```python
from build123d import *

# Parameters (mm, degrees)
SKETCH1_R           = 1.55
SKETCH1_W           = 57.8
SKETCH1_H           = 30
SKETCH1_W_2         = 22
SKETCH1_W_3         = 30
BOSS_EXTRUDE1_DEPTH = 10
FILLET2_R           = 8
CHAMFER1_SIZE       = 1
SKETCH2_R           = 3.25
CUT_EXTRUDE1_DEPTH  = 3
CUT_EXTRUDE2_DEPTH  = 137.363814848
CHAMFER2_SIZE       = 1


with BuildPart() as part:
    # Sketch1 → Boss-Extrude1 (new body)
    # profile 1 of 9: a face of its own
    with BuildSketch(Plane.XY):
        Polygon((-25, -31.5), (-25, -41.5), (25, -41.5), (25, -31.5), (25, -1.5), (25, 8.5), (-25, 8.5), (-25, -1.5), align=None)
        with Locations((0, -33)):
            Circle(SKETCH1_R, mode=Mode.SUBTRACT)
        Circle(SKETCH1_R, mode=Mode.SUBTRACT)
    # profile 2 of 9: a face of its own
    with BuildSketch(Plane.XY):
        with Locations((-53.9, -16.5)):
            Rectangle(SKETCH1_W, SKETCH1_H)
    # profile 3 of 9: a face of its own
    with BuildSketch(Plane.XY):
        with Locations((36, -16.5)):
            Rectangle(SKETCH1_W_2, SKETCH1_H)
    # profile 4 of 9: a face of its own
    with BuildSketch(Plane.XY):
        with Locations((-97.8, -16.5)):
            Rectangle(SKETCH1_W_3, SKETCH1_H)
        with BuildLine():
            Line((-99.8, -24.6), (-99.8, -23.6))
            Line((-99.8, -23.6), (-99.267140075, -23.6))
            ThreePointArc((-99.267140075, -23.6), (-98.896015511, -23.003984489), (-98.3, -22.632859925))
            Line((-98.3, -22.632859925), (-98.3, -22.1))
            Line((-98.3, -22.1), (-97.3, -22.1))
            Line((-97.3, -22.1), (-97.3, -22.632859925))
            ThreePointArc((-97.3, -22.632859925), (-96.703984489, -23.003984489), (-96.332859925, -23.6))
            Line((-96.332859925, -23.6), (-95.8, -23.6))
            Line((-95.8, -23.6), (-95.8, -24.6))
            Line((-95.8, -24.6), (-96.332859925, -24.6))
            ThreePointArc((-96.332859925, -24.6), (-96.703984489, -25.196015511), (-97.3, -25.567140075))
            Line((-97.3, -25.567140075), (-97.3, -26.1))
            Line((-97.3, -26.1), (-98.3, -26.1))
            Line((-98.3, -26.1), (-98.3, -25.567140075))
            ThreePointArc((-98.3, -25.567140075), (-98.896015511, -25.196015511), (-99.267140075, -24.6))
            Line((-99.267140075, -24.6), (-99.8, -24.6))
        make_face(mode=Mode.SUBTRACT)
        with BuildLine():
            Line((-97.3, -10.9), (-98.3, -10.9))
            Line((-98.3, -10.9), (-98.3, -10.367140075))
            ThreePointArc((-98.3, -10.367140075), (-98.896015511, -9.996015511), (-99.267140075, -9.4))
            Line((-99.267140075, -9.4), (-99.8, -9.4))
            Line((-99.8, -9.4), (-99.8, -8.4))
            Line((-99.8, -8.4), (-99.267140075, -8.4))
            ThreePointArc((-99.267140075, -8.4), (-98.896015511, -7.803984489), (-98.3, -7.432859925))
            Line((-98.3, -7.432859925), (-98.3, -6.9))
            Line((-98.3, -6.9), (-97.3, -6.9))
            Line((-97.3, -6.9), (-97.3, -7.432859925))
            ThreePointArc((-97.3, -7.432859925), (-96.703984489, -7.803984489), (-96.332859925, -8.4))
            Line((-96.332859925, -8.4), (-95.8, -8.4))
            Line((-95.8, -8.4), (-95.8, -9.4))
            Line((-95.8, -9.4), (-96.332859925, -9.4))
            ThreePointArc((-96.332859925, -9.4), (-96.703984489, -9.996015511), (-97.3, -10.367140075))
            Line((-97.3, -10.367140075), (-97.3, -10.9))
        make_face(mode=Mode.SUBTRACT)
    # profile 5 of 9: a face of its own
    with BuildSketch(Plane.XY):
        with Locations((62, -16.5)):
            Rectangle(SKETCH1_W_3, SKETCH1_H)
        with BuildLine():
            Line((55.867140075, -23.6), (56.4, -23.6))
            Line((56.4, -23.6), (56.4, -24.6))
            Line((56.4, -24.6), (55.867140075, -24.6))
            ThreePointArc((55.867140075, -24.6), (55.496015511, -25.196015511), (54.9, -25.567140075))
            Line((54.9, -25.567140075), (54.9, -26.1))
            Line((54.9, -26.1), (53.9, -26.1))
            Line((53.9, -26.1), (53.9, -25.567140075))
            ThreePointArc((53.9, -25.567140075), (53.303984489, -25.196015511), (52.932859925, -24.6))
            Line((52.932859925, -24.6), (52.4, -24.6))
            Line((52.4, -24.6), (52.4, -23.6))
            Line((52.4, -23.6), (52.932859925, -23.6))
            ThreePointArc((52.932859925, -23.6), (53.303984489, -23.003984489), (53.9, -22.632859925))
            Line((53.9, -22.632859925), (53.9, -22.1))
            Line((53.9, -22.1), (54.9, -22.1))
            Line((54.9, -22.1), (54.9, -22.632859925))
            ThreePointArc((54.9, -22.632859925), (55.496015511, -23.003984489), (55.867140075, -23.6))
        make_face(mode=Mode.SUBTRACT)
        with BuildLine():
            Line((67.6, -24.6), (67.6, -23.6))
            Line((67.6, -23.6), (68.132859925, -23.6))
            ThreePointArc((68.132859925, -23.6), (68.503984489, -23.003984489), (69.1, -22.632859925))
            Line((69.1, -22.632859925), (69.1, -22.1))
            Line((69.1, -22.1), (70.1, -22.1))
            Line((70.1, -22.1), (70.1, -22.632859925))
            ThreePointArc((70.1, -22.632859925), (70.696015511, -23.003984489), (71.067140075, -23.6))
            Line((71.067140075, -23.6), (71.6, -23.6))
            Line((71.6, -23.6), (71.6, -24.6))
            Line((71.6, -24.6), (71.067140075, -24.6))
            ThreePointArc((71.067140075, -24.6), (70.696015511, -25.196015511), (70.1, -25.567140075))
            Line((70.1, -25.567140075), (70.1, -26.1))
            Line((70.1, -26.1), (69.1, -26.1))
            Line((69.1, -26.1), (69.1, -25.567140075))
            ThreePointArc((69.1, -25.567140075), (68.503984489, -25.196015511), (68.132859925, -24.6))
            Line((68.132859925, -24.6), (67.6, -24.6))
        make_face(mode=Mode.SUBTRACT)
        with BuildLine():
            Line((56.4, -8.4), (56.4, -9.4))
            Line((56.4, -9.4), (55.867140075, -9.4))
            ThreePointArc((55.867140075, -9.4), (55.496015511, -9.996015511), (54.9, -10.367140075))
            Line((54.9, -10.367140075), (54.9, -10.9))
            Line((54.9, -10.9), (53.9, -10.9))
            Line((53.9, -10.9), (53.9, -10.367140075))
            ThreePointArc((53.9, -10.367140075), (53.303984489, -9.996015511), (52.932859925, -9.4))
            Line((52.932859925, -9.4), (52.4, -9.4))
            Line((52.4, -9.4), (52.4, -8.4))
            Line((52.4, -8.4), (52.932859925, -8.4))
            ThreePointArc((52.932859925, -8.4), (53.303984489, -7.803984489), (53.9, -7.432859925))
            Line((53.9, -7.432859925), (53.9, -6.9))
            Line((53.9, -6.9), (54.9, -6.9))
            Line((54.9, -6.9), (54.9, -7.432859925))
            ThreePointArc((54.9, -7.432859925), (55.496015511, -7.803984489), (55.867140075, -8.4))
            Line((55.867140075, -8.4), (56.4, -8.4))
        make_face(mode=Mode.SUBTRACT)
        with BuildLine():
            Line((70.1, -10.9), (69.1, -10.9))
            Line((69.1, -10.9), (69.1, -10.367140075))
            ThreePointArc((69.1, -10.367140075), (68.503984489, -9.996015511), (68.132859925, -9.4))
            Line((68.132859925, -9.4), (67.6, -9.4))
            Line((67.6, -9.4), (67.6, -8.4))
            Line((67.6, -8.4), (68.132859925, -8.4))
            ThreePointArc((68.132859925, -8.4), (68.503984489, -7.803984489), (69.1, -7.432859925))
            Line((69.1, -7.432859925), (69.1, -6.9))
            Line((69.1, -6.9), (70.1, -6.9))
            Line((70.1, -6.9), (70.1, -7.432859925))
            ThreePointArc((70.1, -7.432859925), (70.696015511, -7.803984489), (71.067140075, -8.4))
            Line((71.067140075, -8.4), (71.6, -8.4))
            Line((71.6, -8.4), (71.6, -9.4))
            Line((71.6, -9.4), (71.067140075, -9.4))
            ThreePointArc((71.067140075, -9.4), (70.696015511, -9.996015511), (70.1, -10.367140075))
            Line((70.1, -10.367140075), (70.1, -10.9))
        make_face(mode=Mode.SUBTRACT)
    # profile 6 of 9: a face of its own
    with BuildSketch(Plane.XY):
        with BuildLine():
            Line((77, -31.5), (47, -31.5))
            ThreePointArc((47, -31.5), (62, -46.5), (77, -31.5))
        make_face()
    # profile 7 of 9: a face of its own
    with BuildSketch(Plane.XY):
        with BuildLine():
            ThreePointArc((-112.8, -1.5), (-127.8, -16.5), (-112.8, -31.5))
            Line((-112.8, -31.5), (-112.8, -1.5))
        make_face()
    # profile 8 of 9: a face of its own
    with BuildSketch(Plane.XY):
        with BuildLine():
            ThreePointArc((77, -1.5), (62, 13.5), (47, -1.5))
            Line((47, -1.5), (77, -1.5))
        make_face()
    # profile 9 of 9: a face of its own
    with BuildSketch(Plane.XY):
        with BuildLine():
            Line((77, -1.5), (77, -31.5))
            ThreePointArc((77, -31.5), (92, -16.5), (77, -1.5))
        make_face()
    extrude(amount=BOSS_EXTRUDE1_DEPTH)

    # Fillet2
    fillet2_edges = [part.edges().sort_by_distance(p)[0] for p in [
        (-25, -1.5, 5),
        (25, -1.5, 5),
        (25, -31.5, 5),
        (-25, -31.5, 5),
    ]]
    fillet(fillet2_edges, radius=FILLET2_R)

    # Chamfer1
    chamfer1_edges = [part.edges().sort_by_distance(p)[0] for p in [
        (-127.8, -16.5, 10),
        (-72.9, -1.5, 0),
        (0, 8.5, 0),
        (40, -1.5, 0),
        (62, 13.5, 0),
        (92, -16.5, 0),
        (62, -46.5, 0),
        (40, -31.5, 0),
        (25, -40.5, 0),
        (0, -41.5, 0),
        (-25, -40.5, 0),
        (-72.9, -31.5, 0),
        (-127.8, -16.5, 0),
        (-72.9, -31.5, 10),
        (-25, -40.5, 10),
        (0, -41.5, 10),
        (25, 7.5, 0),
        (25, 7.5, 10),
        (-25, 7.5, 0),
        (-25, 7.5, 10),
        (27.343145751, 0.843145751, 0),
        (27.343145751, 0.843145751, 10),
        (27.343145751, -33.843145751, 0),
        (27.343145751, -33.843145751, 10),
        (25, -40.5, 10),
        (-27.343145751, -33.843145751, 0),
        (-27.343145751, -33.843145751, 10),
        (-27.343145751, 0.843145751, 0),
        (-27.343145751, 0.843145751, 10),
        (40, -31.5, 10),
        (62, -46.5, 10),
        (92, -16.5, 10),
        (62, 13.5, 10),
        (40, -1.5, 10),
        (0, 8.5, 10),
        (-72.9, -1.5, 10),
    ]]
    chamfer(chamfer1_edges, length=CHAMFER1_SIZE)

    # Sketch2 → Cut-Extrude1 (cut)
    with BuildSketch(Plane(origin=(0, 0, 0), x_dir=(-1, 0, 0), z_dir=(0, 0, -1))):
        Circle(SKETCH2_R)
        with Locations((0, -33)):
            Circle(SKETCH2_R)
    extrude(amount=-CUT_EXTRUDE1_DEPTH, mode=Mode.SUBTRACT)

    # Sketch3 → Cut-Extrude2 (cut, through all)
    with BuildSketch(Plane.XY.offset(10)):
        with BuildLine():
            Line((-84.5, -8), (40.5, -8))
            ThreePointArc((40.5, -8), (49, -16.5), (40.5, -25))
            Line((40.5, -25), (-84.5, -25))
            ThreePointArc((-84.5, -25), (-93, -16.5), (-84.5, -8))
        make_face()
    extrude(amount=-CUT_EXTRUDE2_DEPTH, mode=Mode.SUBTRACT)

    # Chamfer2
    chamfer2_edges = [part.edges().sort_by_distance(p)[0] for p in [
        (-93, -16.5, 0),
        (-22, -8, 0),
        (49, -16.5, 0),
        (-22, -25, 0),
        (-93, -16.5, 10),
        (-22, -25, 10),
        (49, -16.5, 10),
        (-22, -8, 10),
    ]]
    chamfer(chamfer2_edges, length=CHAMFER2_SIZE)


solid = part.part
```
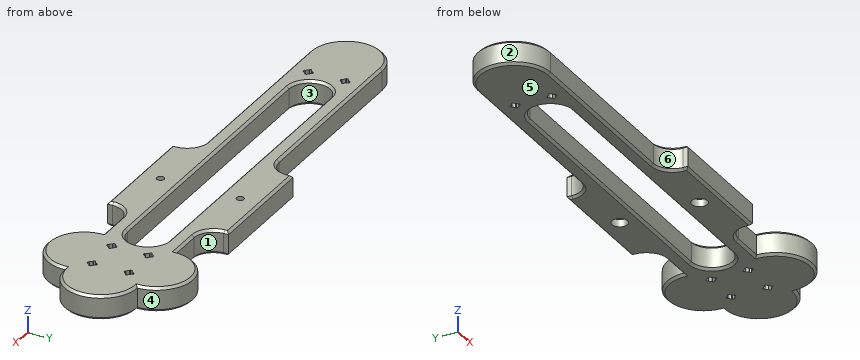
Part model, mm, in its own coordinate system. Face numbers are marked on the shaded views. A direction names the side the tool comes from. Round coordinates to 2 decimals unless told otherwise and drop trailing zeros. Order: outer loops, then holes, each group sorted by start corner. A loop starts at its lowest first (then second) coordinate and runs counter-clockwise, first axis right, second up. Notation, with made-up numbers: M -34,51.25 L -14,51.25 A31 cw -14,88.25 Z; hole C -30,32.25 d1. An arc over 180 degrees is marked long. Answer in a Markdown table with one row per item. Add a question column.
Q1. Mould opens along X. For the marked faces 4, 5 and 6 say: +X half, -X half, draft (parallel to the pull), parting line (faces both ways), or undercut.
Q2. Cut at A-A on x = -105. Give the cut face in (y, z).
Q3. 3-axis set-ups, long thin cutter, end or side, ignore diameter. For the marked faces 1, 2 and 3: which of +Z, -Z, +X, -X, +Y, -Y reach the whole face in a straight line?
Q4. Pin check, flat tips, straight feed: pin 1 (0.6 mm diameter, centred on x = -96, z = 5.5, fed in from +Y); pin 2 (4 mm diameter, centred on x = -4, z = 5.5, fed in from -Y); pin 3 (2 mm diameter, centred on y = 4.5, z = 6.5, fed in from -X). Stop position of each tip, or through.
Q5. Wall check: L1, parallel to Y at x = 0, z = 1.25; L2, parallel to Y at x = 0, z = 5.75; L3, parallel to Y at x = 56, z = 5.75. Give the ranges that are in metal, low to high. Write a range as from..to.
Q6. Cut at B-B on z = 5.25. Give the number of separate pieces and of enclosed holes in the cut face, and give its area (3 significant figures).
Established:
| question | item | result |
|---|---|---|
| 1 | face 4 | undercut |
| 1 | face 5 | draft |
| 1 | face 6 | -X half |
| 2 | outline | M -31.5,1 L -30.5,0 L -2.5,0 L -1.5,1 L -1.5,9 L -2.5,10 L -30.5,10 L -31.5,9 Z |
| 3 | face 1 | +Z, -Z, +Y |
| 3 | face 2 | +Z, -Z, -X |
| 3 | face 3 | +Z, -Z |
| 4 | pin 1 | stops at y = -1.5 |
| 4 | pin 2 | stops at y = -41.5 |
| 4 | pin 3 | stops at x = -25.58 |
| 5 | L1 | y = -41.5..-36.25, -29.75..-25, -8..-3.25, 3.25..8.5 |
| 5 | L2 | y = -41.5..-34.55, -31.45..-25, -8..-1.55, 1.55..8.5 |
| 5 | L3 | y = -45.25..-24.6, -23.6..-9.4, -8.4..12.25 |
| 6 | separate pieces | 1 |
| 6 | enclosed holes | 9 |
| 6 | area | 5,740 mm2 |
